Check sheet for the modelled part. Datum: model origin and axes. Units: mm. A direction names the side the tool comes from. Give positions to 0.01 mm unless a question says otherwise; leave off trailing zeros. Write each loop counter-clockwise with the first axis right and the second up, starting at its lowest first coordinate (ties: lowest second). Pieces come first, ordered by that corner, then holes. Notation, with made-up numbers: (74.25, 21.5) -> (92.25, 21.5) arc R22 cw to (92.25, 42.5) -> close; hole circle Ø2 at (13, 49.5). An arc over 180 degrees is marked (long way). Answer as a JSON object with one key per item and string values.
from build123d import *

# Parameters (mm, degrees)
F1_DEPTH = 12
F2_W     = 11
F2_H     = 2
F3_DEPTH = 15
F4_R     = 1
F5_DEPTH = 7.001
F6_R     = 1
F7_DEPTH = 35.820805


with BuildPart() as f1:
    # F0 (on Front) → F1 (new body)
    with BuildSketch(Plane.XZ):
        Polygon((-64.93865, 4), (-64.93865, 0), (8.06135, 0), (39.881155, -31.819805), (42.7677, -29.049495), (9.718204, 4), align=None)
    extrude(amount=F1_DEPTH)

    # F2 (on face) → F3 (join)
    with BuildSketch(Plane.XY.offset(4)):
        with Locations((-0.281796, -6)):
            Rectangle(F2_W, F2_H)
    extrude(amount=F3_DEPTH)

    # F4 (on face) → F5 (cut, through all)
    with BuildSketch(Plane(origin=(0, -5, 0), x_dir=(-1, 0, 0), z_dir=(0, 1, 0))):
        with Locations((0.281796, 14)):
            Circle(F4_R)
    extrude(amount=-F5_DEPTH, mode=Mode.SUBTRACT)

    # F6 (on face) → F7 (cut, through all)
    with BuildSketch(Plane.XY.offset(4)):
        with Locations((-58.93865, -6)):
            Circle(F6_R)
    extrude(amount=-F7_DEPTH, mode=Mode.SUBTRACT)


solid = f1.part
1. Sectioned sample at B-B, the plane z = 14. Enter the section's corners in (x, y), plus the area to 3 significant figures.
Determined:
{"outline": "(-5.78, -7) -> (-1.28, -7) -> (-1.28, -5) -> (-5.78, -5) -> close; (0.72, -7) -> (5.22, -7) -> (5.22, -5) -> (0.72, -5) -> close", "area": "18.0 mm^2"}
2. Go/stop test with flat-tipped pins: P1, Ø1, axis at y = -6, z = 13.5, coming from the -X side; P2, Ø1, axis at y = -9.5, z = -9, coming from the +X side; P3, Ø6, axis at x = -14, y = -10, coming from the -Z side. Record where each tip stops, or that it passes through.
Determined:
{"P1": "x = -5.78", "P2": "x = 23.22", "P3": "z = 0"}
3. Sectioned sample at D-D, the plane z = -2.5. Enter the section's corners in (x, y).
Determined:
{"outline": "(10.56, -12) -> (16.22, -12) -> (16.22, 0) -> (10.56, 0) -> close"}
4. Sectioned sample at A-A, the plane y = -6. Enter the section's corners in (x, z).
Determined:
{"outline": "(-64.94, 0) -> (-59.94, 0) -> (-59.94, 4) -> (-64.94, 4) -> close; (-57.94, 0) -> (8.06, 0) -> (39.88, -31.82) -> (42.77, -29.05) -> (9.72, 4) -> (5.22, 4) -> (5.22, 19) -> (-5.78, 19) -> (-5.78, 4) -> (-57.94, 4) -> close; hole circle Ø2 at (-0.28, 14)"}
5. Scan lines: L1, parallel to Z at x = -8.5, y = -3.75; L2, parallel to X at y = -3, z = 2; L3, parallel to X at y = -2.5, z = -13.5. Record each from-to range of solid material in increasing order. Write a range as [from, to].
Determined:
{"L1": "[0, 4]", "L2": "[-64.94, 11.72]", "L3": "[21.56, 27.22]"}
6. Access from +Z, -Z, +X, -X, +Y, -Y to the whole of each face (thin tool, end or side, straight path). Record for faces 1 (the face through (-29, -6, 0)), 2 (the face through (0, -5, 11)), 3 (the face through (5.218, -6, 11)).
Determined:
{"face 1": "-Z, -X, +Y, -Y", "face 2": "+Z, +X, -X, +Y", "face 3": "+Z, +X, +Y, -Y"}
7. Sectioned sample at C-C, the plane x = -41.5. Enter the section's corners in (y, z).
Determined:
{"outline": "(-12, 0) -> (0, 0) -> (0, 4) -> (-12, 4) -> close"}
8. Mould release check, pull along Z, two halves, no side actions. Record for faces 4 (the face through (0, -6, 19)), 5 (the face through (-0.065, -5.986, 13.024)), 6 (the face through (41.304, -5.916, -30.454)): released by +Z, released by -Z, zero draft, split by the parting line, or undercut.
Determined:
{"face 4": "released by +Z", "face 5": "undercut", "face 6": "released by -Z"}
